The model under review builds one solid part; all positions refer to its coordinate system, in mm. Face numbers are marked on the shaded views. Round coordinates to 2 decimals unless told otherwise and drop trailing zeros. Order: outer loops, then holes, each group sorted by start corner. A loop starts at its lowest first (then second) coordinate and runs counter-clockwise, first axis right, second up. Notation, with made-up numbers: M 13,15 L 65,15 A17 ccw 65,37 Z; hole C 72.5,11 d11. An arc over 180 degrees is marked long. Answer as CSV lines item,"result". Start each with the question number.
from build123d import *

# Parameters (mm, degrees)
F0_W     = 98.425
F0_H     = 25.4
F1_DEPTH = 1.5875
F3_DEPTH = 1.5875
F6_DEPTH = 1.5875
F5_ANGLE = -90


with BuildPart() as f1:
    # F0 (on Front) → F1 (new body)
    with BuildSketch(Plane.XZ):
        with Locations((49.2125, 12.7)):
            Rectangle(F0_W, F0_H)
    extrude(amount=F1_DEPTH)

    # F2 (on face) → F3 (join)
    with BuildSketch(Plane.XZ.offset(1.5875)):
        Polygon((21.4400661804, 23.01875), (9.525, 2.38125), (28.575, 2.38125), (40.4900661804, 23.01875), align=None)
        Polygon((42.0775661804, 23.01875), (30.1625, 2.38125), (37.30625, 2.38125), (42.0775661804, 10.6454120434), (42.0775661804, 2.38125), (49.2213161804, 2.38125), (53.9926323608, 10.6454120434), (53.9926323608, 2.38125), (61.1363823608, 2.38125), (61.1363823608, 23.01875), (53.9926323608, 23.01875), (49.2213161804, 14.7545879566), (49.2213161804, 23.01875), align=None)
        with BuildLine():
            ThreePointArc((66.6397834492, 22.6730891893), (66.1129825156, 22.4233597915), (65.8988823608, 21.8811005183))
            Line((65.8988823608, 21.8811005183), (65.8988823608, 17.859375))
            ThreePointArc((65.8988823608, 17.859375), (66.1313663532, 17.2981089924), (66.6926323608, 17.065625))
            Line((66.6926323608, 17.065625), (72.2488823608, 17.065625))
            Line((72.2488823608, 17.065625), (72.2488823608, 18.25625))
            ThreePointArc((72.2488823608, 18.25625), (72.4813663532, 18.8175160076), (73.0426323608, 19.05))
            Line((73.0426323608, 19.05), (80.9801323608, 19.05))
            ThreePointArc((80.9801323608, 19.05), (81.5413983684, 18.8175160076), (81.7738823608, 18.25625))
            Line((81.7738823608, 18.25625), (81.7738823608, 15.478125))
            ThreePointArc((81.7738823608, 15.478125), (81.5413983684, 14.9168589924), (80.9801323608, 14.684375))
            Line((80.9801323608, 14.684375), (72.2488823608, 14.684375))
            Line((72.2488823608, 14.684375), (72.2488823608, 10.715625))
            Line((72.2488823608, 10.715625), (80.9801323608, 10.715625))
            ThreePointArc((80.9801323608, 10.715625), (81.5413983684, 10.4831410076), (81.7738823608, 9.921875))
            Line((81.7738823608, 9.921875), (81.7738823608, 7.14375))
            ThreePointArc((81.7738823608, 7.14375), (81.5413983684, 6.5824839924), (80.9801323608, 6.35))
            Line((80.9801323608, 6.35), (73.0426323608, 6.35))
            ThreePointArc((73.0426323608, 6.35), (72.4813663532, 6.5824839924), (72.2488823608, 7.14375))
            Line((72.2488823608, 7.14375), (72.2488823608, 8.334375))
            Line((72.2488823608, 8.334375), (66.6926323608, 8.334375))
            ThreePointArc((66.6926323608, 8.334375), (66.1313663532, 8.1018910076), (65.8988823608, 7.540625))
            Line((65.8988823608, 7.540625), (65.8988823608, 3.5188994817))
            ThreePointArc((65.8988823608, 3.5188994817), (66.1129825156, 2.9766402085), (66.6397834492, 2.7269108107))
            ThreePointArc((66.6397834492, 2.7269108107), (77.0113823608, 2.38125), (87.3829812725, 2.7269108107))
            ThreePointArc((87.3829812725, 2.7269108107), (87.909782206, 2.9766402085), (88.1238823608, 3.5188994817))
            Line((88.1238823608, 3.5188994817), (88.1238823608, 11.90625))
            ThreePointArc((88.1238823608, 11.90625), (87.8913983684, 12.4675160076), (87.3301323608, 12.7))
            ThreePointArc((87.3301323608, 12.7), (87.8913983684, 12.9324839924), (88.1238823608, 13.49375))
            Line((88.1238823608, 13.49375), (88.1238823608, 16.8671875))
            Line((88.1238823608, 16.8671875), (88.1238823608, 21.8811005183))
            ThreePointArc((88.1238823608, 21.8811005183), (87.909782206, 22.4233597915), (87.3829812725, 22.6730891893))
            ThreePointArc((87.3829812725, 22.6730891893), (77.0113823608, 23.01875), (66.6397834492, 22.6730891893))
        make_face()
    extrude(amount=F3_DEPTH)

    # F4 (on face) → F6 (cut, through all)
    with BuildSketch(Plane.XZ.offset(3.175)):
        Polygon((22.4234375, 2.38125), (34.3385036804, 23.01875), (33.9416286804, 23.01875), (22.0265625, 2.38125), align=None)
        Polygon((16.0734375, 2.38125), (27.9885036804, 23.01875), (27.5916286804, 23.01875), (15.6765625, 2.38125), align=None)
    extrude(amount=-F6_DEPTH, mode=Mode.SUBTRACT)


with BuildPart() as f1_1:
    # F5: moved
    add(f1.part.rotate(Axis((49.2125, 0, 0), (1, 0, 0)), F5_ANGLE))


solid = f1_1.part
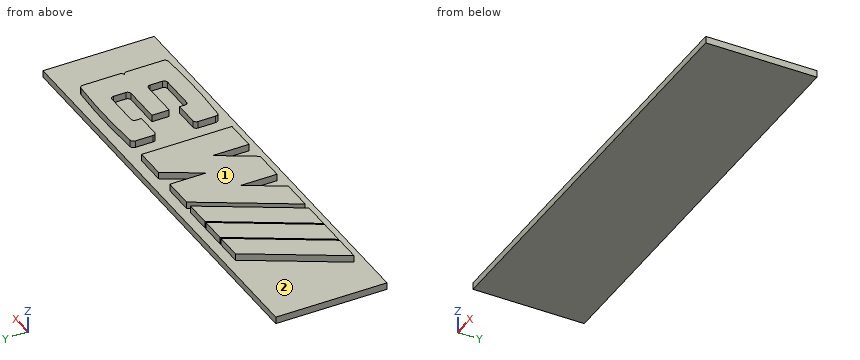
Item 1: Consider section B-B (z = 2.4). State how many separate pieces and enclosed holes the cut face has, and give its area (3 significant figures).
Item 2: Wall thickness on probe 1 along X at (y, z) = (15.25, 1.9); probe 2 along X at (y, z) = (19.5, 2.45); probe 3 along Y at (x, z) = (67.5, 1.8): over which ranges is each line inside the solid? List them lowest first. Write a range as [from, to].
Item 3: For pin 1 (0.5 mm diameter, centred on x = 26.5, z = 2, fed in from -Y); pin 2 (0.6 mm diameter, centred on y = 17.5, z = 2.5, fed in from +X); pin 3 (0.5 mm diameter, centred on x = 36, z = 2, fed in from +Y), all flat-tipped, find the tip position at first contact; note any pin that passes through.
Item 4: Consider section A-A (x = 59). State the section outline as (y, z) points (1 decimal), and give its area (3 significant figures).
Item 5: The part is to be moulded in two halves that separate along X. For the marked faces 1 and 2, say which applies: +X half, -X half, draft (parallel to the pull), parting line (faces both ways), or undercut.
Item 6: Consider section D-D (x = 10.5). State the section outline as (y, z) points (1 decimal), and give its area (3 significant figures).
Reported:
1,separate pieces,"5"
1,enclosed holes,"0"
1,area,"1,150 mm²"
2,probe 1,"x = [16.95, 23.11], [23.5, 29.46], [29.85, 36], [37.59, 49.22], [49.51, 61.14], [81.74, 88.12]"
2,probe 2,"x = [19.41, 25.56], [25.96, 31.91], [32.31, 38.46], [40.05, 49.22], [51.96, 61.14], [65.9, 88.12]"
2,probe 3,"y = [2.67, 8.33], [17.07, 22.73]"
3,pin 1,"stops at y = 2.38"
3,pin 2,"stops at x = 88.12"
3,pin 3,"stops at y = 23.02"
4,outline,"M 0,0 L 25.4,0 L 25.4,1.6 L 23,1.6 L 23,3.2 L 2.4,3.2 L 2.4,1.6 L 0,1.6 Z"
4,area,"73.1 mm²"
5,face 1,"draft"
5,face 2,"undercut"
6,outline,"M 0,0 L 25.4,0 L 25.4,1.6 L 4.1,1.6 L 4.1,3.2 L 2.4,3.2 L 2.4,1.6 L 0,1.6 Z"
6,area,"43.0 mm²"
